Here's how the part is built. I have some questions about the finished solid (model axes, mm). Round coordinates to 2 decimals unless told otherwise and drop trailing zeros. Write each loop counter-clockwise with the first axis right and the second up, starting at its lowest first coordinate (ties: lowest second). Pieces come first, ordered by that corner, then holes. Notation, with made-up numbers: (-36.5, 2.5) -> (4.5, 2.5) arc R17 ccw to (4.5, 17.5) -> close; hole circle Ø2 at (22.5, -30.5). An arc over 180 degrees is marked (long way). Answer as CSV lines item,"result".
```python
from build123d import *

# Parameters (mm, degrees)
SKETCH002_W     = 388.595154
SKETCH002_H     = 392.901
SKETCH002_R     = 1.62754
SKETCH002_R_2   = 1.622912
SKETCH002_R_3   = 1.629974
SKETCH002_R_4   = 1.642619
SKETCH002_R_5   = 1.621975
SKETCH002_R_6   = 1.620988
SKETCH002_R_7   = 1.638708
SKETCH002_R_8   = 1.617701
PAD_DEPTH       = 6.35
POCKET001_DEPTH = 57
SKETCH007_W     = 49.299805
SKETCH007_H     = 32.819429
POCKET_DEPTH    = 69
SKETCH009_R     = 10
POCKET003_DEPTH = 26


with BuildPart() as part:
    # Sketch002 → Pad (new body)
    with BuildSketch(Plane.XY.offset(-307)):
        with Locations((505.886505, 39.199462)):
            Rectangle(SKETCH002_W, SKETCH002_H)
        with Locations((322.359876, -87.178603)):
            Circle(SKETCH002_R, mode=Mode.SUBTRACT)
        with Locations((382.343016, -147.173684)):
            Circle(SKETCH002_R_2, mode=Mode.SUBTRACT)
        with Locations((630.524069, -147.355562)):
            Circle(SKETCH002_R_3, mode=Mode.SUBTRACT)
        with Locations((690.492891, -87.34992)):
            Circle(SKETCH002_R_4, mode=Mode.SUBTRACT)
        with Locations((689.91036, 163.255499)):
            Circle(SKETCH002_R_5, mode=Mode.SUBTRACT)
        with Locations((629.919382, 223.232625)):
            Circle(SKETCH002_R_6, mode=Mode.SUBTRACT)
        with Locations((382.677955, 223.228676)):
            Circle(SKETCH002_R_7, mode=Mode.SUBTRACT)
        with Locations((322.692155, 163.204715)):
            Circle(SKETCH002_R_8, mode=Mode.SUBTRACT)
    extrude(amount=PAD_DEPTH)

    # Sketch004 → Pocket001 (cut)
    with BuildSketch(Plane(origin=(0, 0, -307), x_dir=(1, 0, 0), z_dir=(0, 0, -1))):
        Polygon((484.382596, -177.360658), (484.382596, -211.810965), (488.793788, -216.222157), (523.215023, -216.222157), (527.750201, -211.68698), (527.750201, -177.514144), (523.239443, -173.003385), (488.739868, -173.003385), align=None)
    extrude(amount=-POCKET001_DEPTH, mode=Mode.SUBTRACT)

    # Sketch007 → Pocket (cut)
    with BuildSketch(Plane(origin=(0, 0, -307), x_dir=(1, 0, 0), z_dir=(0, 0, -1))):
        with Locations((506.359008, 9.442521)):
            Rectangle(SKETCH007_W, SKETCH007_H)
    extrude(amount=-POCKET_DEPTH, mode=Mode.SUBTRACT)

    # Sketch009 → Pocket003 (cut)
    with BuildSketch(Plane(origin=(0, 0, -307), x_dir=(1, 0, 0), z_dir=(0, 0, -1))):
        with Locations((393.495178, -177.602295)):
            Circle(SKETCH009_R)
    extrude(amount=-POCKET003_DEPTH, mode=Mode.SUBTRACT)


with BuildPart() as part_1:
    # Body placement: moved
    add(part.part.moved(Location((0, 0, 51))))


solid = part_1.part
```
1. Suppose I cut it at D-D on y = -3. Please give me the cut outline in (x, z).
Numbers:
outline,"(311.59, -256) -> (481.71, -256) -> (481.71, -249.65) -> (311.59, -249.65) -> close; (531.01, -256) -> (700.18, -256) -> (700.18, -249.65) -> (531.01, -249.65) -> close"
2. Suppose I cut it at B-B on y = 193. Please give me the cut outline in (x, z).
Numbers:
outline,"(311.59, -256) -> (484.38, -256) -> (484.38, -249.65) -> (311.59, -249.65) -> close; (527.75, -256) -> (700.18, -256) -> (700.18, -249.65) -> (527.75, -249.65) -> close"
3. If I drill on line 1 (Y direction, x = 510.5, z = -251.75); line 2 (X direction, y = 183.5, z = -255.25), over which ranges is the centre line in solid material (lowest first)?
Numbers:
line 1,"y = -157.25 to -25.85, 6.97 to 173, 216.22 to 235.65"
line 2,"x = 311.59 to 385.42, 401.57 to 484.38, 527.75 to 700.18"
4. If we mould it in two halves opening along Y, with no side actions, what happens to faces 1 (the face through (503, 42, -249.65)), 2 (the face through (402.733, 181.432, -252.869))? For each: released by +Y, released by -Y, zero draft, split by the parting line, or undercut.
Numbers:
face 1,"zero draft"
face 2,"undercut"
5. Suppose I cut it at A-A on x = 501.5. Please give me the cut outline in (y, z).
Numbers:
outline,"(-157.25, -256) -> (-25.85, -256) -> (-25.85, -249.65) -> (-157.25, -249.65) -> close; (6.97, -256) -> (173, -256) -> (173, -249.65) -> (6.97, -249.65) -> close; (216.22, -256) -> (235.65, -256) -> (235.65, -249.65) -> (216.22, -249.65) -> close"
6. Suppose I cut it at C-C on z = -252.5. Count the separate pieces of the cut face and the enclosed holes in it, and give its area (3 significant figures).
Numbers:
separate pieces,"1"
enclosed holes,"11"
area,"149,000 mm^2"
